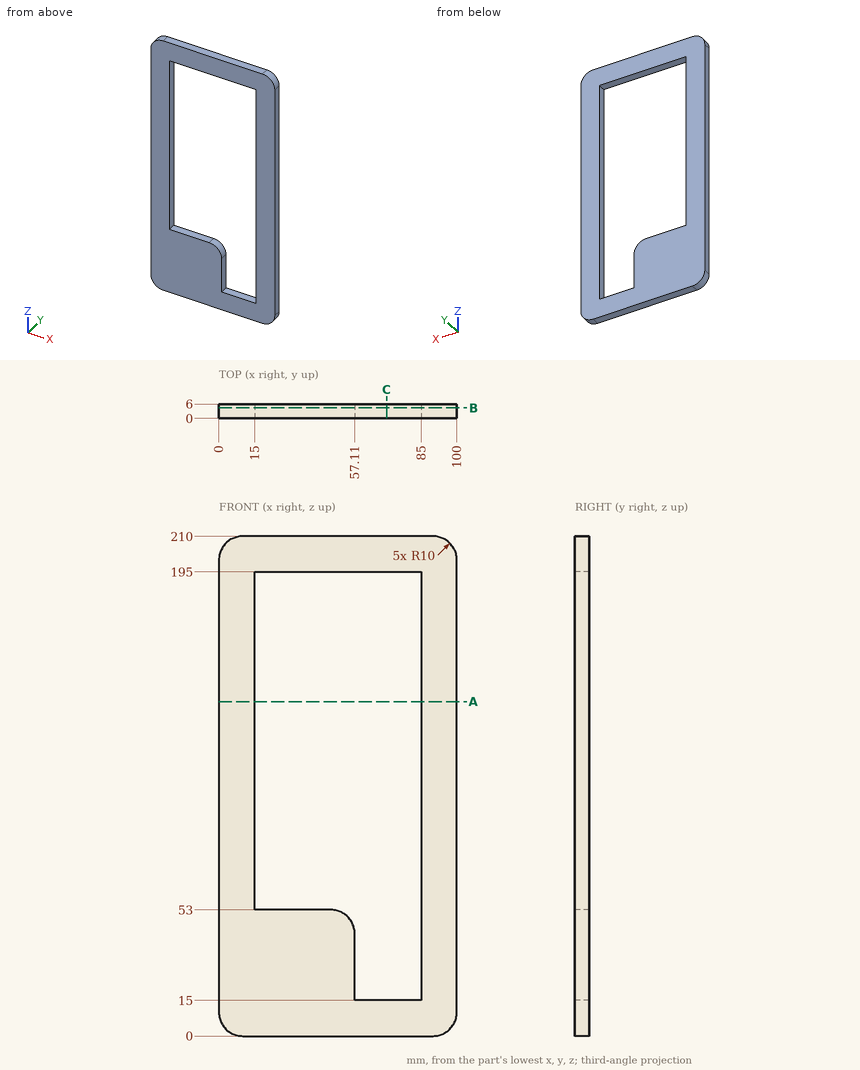
Geometry check sheet. Reference: drawing and pictorial views, mm from the part's lowest x, y, z. Round coordinates to 2 decimals unless told otherwise and drop trailing zeros. Loops run counter-clockwise (first coordinate to the right, second up) from the corner with the lowest first, then second, coordinate; pieces in that order, holes last. Notation, with made-up numbers: (50.5, 60) - (74.5, 60) arc R21 cw to (74.5, 72) - close; hole circle Ø1 at (-24.5, 74.5). An arc over 180 degrees is marked (long way). Use a Markdown table: item, result.
Q1. Cross-section at B-B on y = 4.35. Record the cut outline in (x, z).
Solutions:
| item | result |
|---|---|
| outline | (0, 10) arc R10 ccw to (10, 0) - (90, 0) arc R10 ccw to (100, 10) - (100, 200) arc R10 ccw to (90, 210) - (10, 210) arc R10 ccw to (0, 200) - close; hole (15, 53) - (47.11, 53) arc R10 cw to (57.11, 43) - (57.11, 15) - (85, 15) - (85, 195) - (15, 195) - close |
Q2. Go/stop test with a flat-tipped pin: P1, Ø3, axis at x = 60.5, z = 35.5, coming from the -Y side. Record where the tip stops, or that it passes through.
Solutions:
| item | result |
|---|---|
| P1 | passes through |
Q3. Cross-section at A-A on z = 140.5. Record the cut outline in (x, y).
Solutions:
| item | result |
|---|---|
| outline | (0, 0) - (15, 0) - (15, 6) - (0, 6) - close; (85, 0) - (100, 0) - (100, 6) - (85, 6) - close |
Q4. Cross-section at C-C on x = 70.5. Record the cut outline in (y, z).
Solutions:
| item | result |
|---|---|
| outline | (0, 0) - (6, 0) - (6, 15) - (0, 15) - close; (0, 195) - (6, 195) - (6, 210) - (0, 210) - close |
Q5. Material ranges on line 1 (Z direction, x = 83, y = 3.3); line 2 (X direction, y = 5.15, z = 36); line 3 (Z direction, x = 20, y = 3.4), recorded low to high.
Solutions:
| item | result |
|---|---|
| line 1 | z = 0 to 15, 195 to 210 |
| line 2 | x = 0 to 57.11, 85 to 100 |
| line 3 | z = 0 to 53, 195 to 210 |
